Autodesk Inventor part; units mm, degrees
ref_plane "Work Plane1" through (104.775, 0, 0) normal (0, 0, -1) x (1, 0, 0)
ref_plane "YZ Plane" through (0, 0, 0) normal (1, 0, 0) x (0, 1, 0)
ref_plane "XZ Plane" through (0, 0, 0) normal (0, 1, 0) x (-1, 0, 0)
sketch "Sketch1" plane through (0, 0, 0) normal (0, 0, 1) x (1, 0, 0)
  line L0 (22, 0) -> (22, 2.5)
  line L1 (22, 2.5) -> (12, 2.5)
  line L2 (12, 2.5) -> (11.5092, 2.5)
  line L3 (0, 5) -> (0, 1.7321)
  line L4 (0, 1.7321) -> (1.9, 1.7321)
  line L5 (1.9, 1.7321) -> (2.9, 0)
  line L6 (2.9, 0) -> (22, 0)
  line L7 (0, 5) -> (0.5, 5)
  line L8 (0.5, 5) -> (3, 2.5)
  line L9 (11.5092, 2.5) -> (3, 2.5)
  line L10 (12, 2.5) -> (3, 2.5) construction
  line L11 (3, 2.5) -> (3, 2.5)
  line L12 (-4.4, 0) -> (26.4, 0)
  line L13 (0, -1) -> (0, 6)
  dimension "d0" = 22
  dimension "d1" = 10
  dimension "d2" = 1.9
  dimension "d3" = 5
  dimension "d6" = 3
  dimension "d7" = 45
  dimension "d8" = 3.4641
  dimension "d9" = 60
  dimension "d10" = 10
  dimension "d11" = 5
  dimension "d12" = 0.4908
revolve "Body" add sketch "Sketch1" angle 360 about axis through (2.9, 0, 0) along (1, 0, 0) contours L6 L5 L4 L3 L7 L8 L9 L2 L1 L0
sketch "Sketch2" plane through (0, 0, 0) normal (-1, 0, 0) x (0, 0, 1)
  circle A0 centre (0, 0) radius 1.7321
  line L0 (0, -7) -> (0, 7)
  line L1 (-7, 0) -> (7, 0)
  line L2 (1.7321, 0) -> (0.866, -1.5)
  line L3 (0.866, -1.5) -> (-0.866, -1.5)
  line L4 (-0.866, -1.5) -> (-1.7321, 0)
  line L5 (-1.7321, 0) -> (-0.866, 1.5)
  line L6 (-0.866, 1.5) -> (0.866, 1.5)
  line L7 (0.866, 1.5) -> (1.7321, 0)
  point P0 (0, 1.7321)
extrude "Slot" add sketch "Sketch2" against normal up to next contours L7 A0 | A0 L2 | L6 L0 A0 | A0 L0 L3 | L0 L6 A0 | A0 L3 L0 | L4 A0 | A0 L5
thread "Thread"
chamfer "Chamfer1" distance 0.5112 distance2 0.4908 1 edges at (22, -2.5, 0) measured on face at (22, 0.4809, 1.1324)
ref_plane "Work Plane1" through (104.775, 0, 0) normal (0, 0, -1) x (1, 0, 0)
equation "\"d15\" = GEL"
equation "\"d17\" = -0.5 * SPD + 0.5 * GD"
equation "\"d18\" = GUL"
equation "\"d2\" = INTI"
equation "\"d3\" = GD"
equation "\"d7\" = 0.5 * SEWI"
equation "\"d8\" = 1.1547 * SW"
equation "\"d11\" = BDM"
equation "\"d12\" = GAL"
equation "\"INTI\" = 1.9"
equation "\"GEL\" = 22"
equation "\"GAL\" = 0.61345 * PTC"
equation "\"KOH\" = 3.1"
equation "\"KOD\" = 9.75"
equation "\"GUL\" = 0.61345 * PTC"
equation "\"SPD\" = 3.97758"
equation "\"BDM\" = NND"
equation "\"GD\" = NND"
equation "\"SEWI\" = 90deg"
equation "\"SW\" = 3"
equation "\"TOA\" = 30deg"
equation "\"GD1\" = THREADDIA - 1.2269 * PTC"
equation "\"EPV\" = 4.875"
equation "\"THREADDIA\" = 5"
equation "\"PTC\" = 0.8"
equation "\"NND\" = 5"
equation "\"E0\" = 1.155 * SW"
properties part number "ANSI/IFI 535 - M5x0.8 x 40, FHSFCHCSM" material "Steel, Mild"
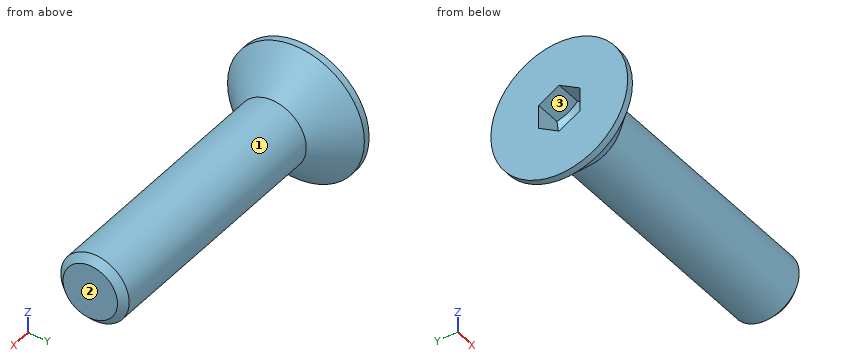
Can you work these out from the model? Positions are in its coordinate system, mm. Face numbers are marked on the shaded views. Coordinates: 2 decimals unless noted, no trailing zeros. Write each loop counter-clockwise with the first axis right and the second up, starting at its lowest first coordinate (ties: lowest second). Pieces come first, ordered by that corner, then holes. Notation, with made-up numbers: M -4.75,-17 L 39.25,-17 A35 ccw 39.25,21 Z; hole C 18,23.25 d3. An arc over 180 degrees is marked long. Use one line per item in the form item = value.
Q1. I need wall thicknesses on line 1 along Z through (x, y) = (16.25, -0.25); line 2 along X through (y, z) = (-3.25, 1.5); line 3 along Z through (x, y) = (10.25, 1.5). Which ranges of each line are inside material? Lowest first, please. Write a range as from..to.
Model answer:
line_1 = -2.49..2.49
line_2 = 0..1.92
line_3 = -2..2
Q2. If we section it at A-A (x = 12.75): Write out the boundary of the cut face in (y, z).
Model answer:
outline = C 0,0 d5
Q3. We'd pull the mould along Y, two halves only. Please class the marked faces 1, 2 and 3: +Y half, -Y half, draft (parallel to the pull), parting line (faces both ways), or undercut.
Model answer:
face_1 = parting line
face_2 = draft
face_3 = undercut
Q4. For P1, Ø4, axis at x = 11, y = -3.5, coming from the -Z side; P2, Ø6, axis at x = 19.5, z = 2, coming from the -Y side; P3, Ø3, axis at x = 3.5, y = 0, coming from the -Z side, each with a flat end and sliding along its axis, tell me the tip position at first contact or that it passes through.
Model answer:
P1 = -2
P2 = -2.5
P3 = -3.5
